Read the model definition and answer for the solid it produces. Units are mm, in the model's axes. Coordinates: 2 decimals unless noted, no trailing zeros. Write each loop counter-clockwise with the first axis right and the second up, starting at its lowest first coordinate (ties: lowest second). Pieces come first, ordered by that corner, then holes. Notation, with made-up numbers: (-23.5, 38.25) -> (-9.5, 38.25) arc R26 ccw to (-9.5, 61.25) -> close; hole circle Ø3 at (16.5, 83.25). An arc over 180 degrees is marked (long way). Use CSV: the item, a comma, the result in double quotes.
from build123d import *

# Parameters (mm, degrees)
BOSS_EXTRUDE1_DEPTH = 10.16
SKETCH5_W           = 63.5
SKETCH5_H           = 20.32
CUT_EXTRUDE1_DEPTH  = 11.16


with BuildPart() as part:
    # Sketch1 → Boss-Extrude1 (new body)
    with BuildSketch(Plane.XY):
        Polygon((-123.444, 2072.64), (-205.715298803, 2072.64), (-205.715298803, 2052.32), (-215.881789204, 2052.32), (-215.881789204, 1963.42), (-205.715298803, 1963.42), (-205.715298803, 1874.52), (-215.881789204, 1874.52), (-215.881789204, 1785.62), (-205.715298803, 1785.62), (-205.715298803, 1696.72), (-215.875298803, 1696.72), (-215.875298803, 1607.82), (-205.715298803, 1607.82), (-205.715298803, 1518.92), (-215.881789204, 1518.92), (-215.881789204, 1488.440000035), (-533.381789204, 1488.440000035), (-533.381789204, 0), (-375.428294602, 0), (-375.428294602, 20.32), (-280.9748, 20.32), (-280.9748, 0), (280.9748, 0), (280.9748, 20.32), (375.428294602, 20.32), (375.428294602, 0), (533.381789204, 0), (533.381789204, 1488.440000035), (215.881789204, 1488.440000035), (215.881789204, 1518.92), (205.715298803, 1518.92), (205.715298803, 1607.82), (215.875298803, 1607.82), (215.875298803, 1696.72), (205.715298803, 1696.72), (205.715298803, 1785.62), (215.881789204, 1785.62), (215.881789204, 1874.52), (205.715298803, 1874.52), (205.715298803, 1963.42), (215.881789204, 1963.42), (215.881789204, 2052.32), (205.715298803, 2052.32), (205.715298803, 2072.64), (123.444, 2072.64), (123.444, 2052.32), (41.135649402, 2052.32), (41.135649402, 2072.64), (-41.135649402, 2072.64), (-41.135649402, 2052.32), (-123.444, 2052.32), align=None)
        Polygon((215.881789204, 1463.040000035), (222.040744894, 1374.366931824), (211.92306481, 1373.664189215), (205.715298803, 1463.040000035), align=None, mode=Mode.SUBTRACT)
        Polygon((-205.715298803, 1463.040000035), (-211.92306481, 1373.664189215), (-222.040744894, 1374.366931824), (-215.881789204, 1463.040000035), align=None, mode=Mode.SUBTRACT)
        Polygon((227.836927701, 1290.916856945), (234.358656272, 1197.020795404), (224.240976188, 1196.318052795), (217.719247617, 1290.214114336), align=None, mode=Mode.SUBTRACT)
        Polygon((-308.266124544, 132.94397688), (-301.755453134, 226.680843836), (-291.63777305, 225.978101227), (-298.14844446, 132.241234271), align=None, mode=Mode.SUBTRACT)
        Polygon((-289.435698895, 404.053512688), (-279.318018811, 403.350770078), (-285.830533081, 309.587370692), (-295.948213166, 310.290113301), align=None, mode=Mode.SUBTRACT)
        Polygon((-283.630301787, 487.636249721), (-277.115944656, 581.426181539), (-266.998264572, 580.72343893), (-273.512621703, 486.933507112), align=None, mode=Mode.SUBTRACT)
        Polygon((-264.796190418, 758.798850391), (-254.678510334, 758.096107781), (-261.194710324, 664.279643533), (-271.312390408, 664.982386142), align=None, mode=Mode.SUBTRACT)
        Polygon((-252.476436179, 936.171519242), (-242.358756095, 935.468776633), (-248.876798945, 841.625779953), (-258.99447903, 842.328522563), align=None, mode=Mode.SUBTRACT)
        Polygon((301.755453134, 226.680843836), (308.266124544, 132.94397688), (298.14844446, 132.241234271), (291.63777305, 225.978101227), align=None, mode=Mode.SUBTRACT)
        Polygon((279.318018811, 403.350770078), (289.435698895, 404.053512688), (295.948213166, 310.290113301), (285.830533081, 309.587370692), align=None, mode=Mode.SUBTRACT)
        Polygon((254.678510334, 758.096107781), (264.796190418, 758.798850391), (271.312390408, 664.982386142), (261.194710324, 664.279643533), align=None, mode=Mode.SUBTRACT)
        Polygon((242.358756095, 935.468776633), (252.476436179, 936.171519242), (258.99447903, 842.328522563), (248.876798945, 841.625779953), align=None, mode=Mode.SUBTRACT)
        Polygon((277.115944656, 581.426181539), (283.630301787, 487.636249721), (273.512621703, 486.933507112), (266.998264572, 580.72343893), align=None, mode=Mode.SUBTRACT)
        Polygon((-240.15668194, 1113.544188093), (-230.039001856, 1112.841445484), (-236.558887567, 1018.971916374), (-246.676567651, 1019.674658983), align=None, mode=Mode.SUBTRACT)
        Polygon((-227.836927701, 1290.916856945), (-217.719247617, 1290.214114336), (-224.240976188, 1196.318052795), (-234.358656272, 1197.020795404), align=None, mode=Mode.SUBTRACT)
        Polygon((230.039001856, 1112.841445484), (240.15668194, 1113.544188093), (246.676567651, 1019.674658983), (236.558887567, 1018.971916374), align=None, mode=Mode.SUBTRACT)
    extrude(amount=BOSS_EXTRUDE1_DEPTH)

    # Sketch5 → Cut-Extrude1 (cut, through all)
    with BuildSketch(Plane.XY.offset(10.16)):
        with Locations((-501.631789204, 10.16)):
            Rectangle(SKETCH5_W, SKETCH5_H)
        with Locations((501.631789204, 10.16)):
            Rectangle(SKETCH5_W, SKETCH5_H)
    extrude(amount=-CUT_EXTRUDE1_DEPTH, mode=Mode.SUBTRACT)


solid = part.part
1. Each of these flat-tipped pins is pushed along its axis until it touches: pin 1 Ø5 at (x, z) = (-345.5, 3.5) entering from -Y; pin 2 Ø3 at (y, z) = (6, 3) entering from -X; pin 3 Ø3 at (y, z) = (11.5, 3) entering from +X. Where does it stop, or does it pass through?
Solutions:
pin 1,"stops at y = 20.32"
pin 2,"stops at x = -469.88"
pin 3,"stops at x = 469.88"
2. A cutting plane is placed at B-B (z = 4). Give the number of separate pieces and of enclosed holes in the cut face, and give its area (3 significant figures).
Solutions:
separate pieces,"1"
enclosed holes,"16"
area,"1,810,000 mm^2"
3. Find the intervals of material crossed by line 1 along X through (y, z) = (1448, 9.25); line 2 along X through (y, z) = (908.5, 7); line 3 along X through (y, z) = (1741.5, 2.75), in increasing order.
Solutions:
line 1,"x = -533.38 to -216.93, -206.76 to 206.76, 216.93 to 533.38"
line 2,"x = -533.38 to -254.4, -244.23 to 244.23, 254.4 to 533.38"
line 3,"x = -205.72 to 205.72"
4. A cutting plane is placed at C-C (x = -400.5). Give the vertices of the cut face in (y, z).
Solutions:
outline,"(0, 0) -> (1488.44, 0) -> (1488.44, 10.16) -> (0, 10.16) -> close"
5. A cutting plane is placed at A-A (y = 1256.5). Give the vertices of the cut face in (x, z).
Solutions:
outline,"(-533.38, 0) -> (-230.23, 0) -> (-230.23, 10.16) -> (-533.38, 10.16) -> close; (-220.06, 0) -> (220.06, 0) -> (220.06, 10.16) -> (-220.06, 10.16) -> close; (230.23, 0) -> (533.38, 0) -> (533.38, 10.16) -> (230.23, 10.16) -> close"
